Verification items for the finished model (mm, model axes). Give positions to 0.01 mm unless a question says otherwise; leave off trailing zeros. Order: outer loops, then holes, each group sorted by start corner. A loop starts at its lowest first (then second) coordinate and runs counter-clockwise, first axis right, second up. Notation, with made-up numbers: (45.5, -9.5) - (99.5, -9.5) arc R34 ccw to (99.5, 26.5) - close; hole circle Ø2 at (-14.5, -22). An arc over 180 degrees is marked (long way). Answer as a JSON object with one key per item and string values.
```python
from build123d import *

# Parameters (mm, degrees)
ESBO_O1_R                = 32
RESSALTO_EXTRUS_O1_DEPTH = 6
FURO_COM_FOLGA_DE_M51_D  = 5.5


with BuildPart() as part:
    # Esboço1 → Ressalto-extrusão1 (new body)
    with BuildSketch(Plane.XY.offset(10)):
        Polygon((16.091018061, 61.251677836), (45, 44.561069332), (45, -44.561069332), (16.091018061, -61.251677836), (-61.091018061, -16.690608504), (-61.091018061, 16.690608504), align=None)
        Circle(ESBO_O1_R, mode=Mode.SUBTRACT)
    extrude(amount=RESSALTO_EXTRUS_O1_DEPTH)

    # Furo com folga de M51 (through all)
    with Locations(Plane(origin=(-55, 0, 16), x_dir=(1, 0, 0), z_dir=(0, 0, 1))):
        with Locations((0, 0), (82.5, 47.631397208), (82.5, -47.631397208)):
            Hole(FURO_COM_FOLGA_DE_M51_D / 2)


solid = part.part
```
(1) Section check C-C (y = 21). Record the cut outline in (x, z).
Computed values:
{"outline": "(-53.63, 10) - (-24.15, 10) - (-24.15, 16) - (-53.63, 16) - close; (24.15, 10) - (45, 10) - (45, 16) - (24.15, 16) - close"}
(2) Gauge pin test, flat ends, axial feed: pin 1 Ø1 at (y, z) = (-30.5, 14) entering from -X; pin 2 Ø1.5 at (y, z) = (-24.5, 11) entering from -X. Record the tip position at first contact, or that the pin passes through.
Computed values:
{"pin 1": "stops at x = -38.04", "pin 2": "stops at x = -48.86"}
(3) Release check for a two-part mould opening along X. For faces 1 (the cylindrical face through (29.682, -49.305, 12.958)), 2 (the flat face through (45, 1, 13)), 3 (the flat face through (-19, -26, 10)) record: pulls with the +X half, pulls with the -X half, needs draft (parallel to the pull), parting line crosses it, or undercut.
Computed values:
{"face 1": "undercut", "face 2": "pulls with the +X half", "face 3": "needs draft"}
(4) Section check A-A (y = 0). Record the cut outline in (x, z).
Computed values:
{"outline": "(-61.09, 10) - (-57.75, 10) - (-57.75, 16) - (-61.09, 16) - close; (-52.25, 10) - (-32, 10) - (-32, 16) - (-52.25, 16) - close; (32, 10) - (45, 10) - (45, 16) - (32, 16) - close"}
(5) Section check D-D (z = 14.5). Record the cut outline in (x, y), then the cut area to 3 significant figures.
Computed values:
{"outline": "(-61.09, -16.69) - (16.09, -61.25) - (45, -44.56) - (45, 44.56) - (16.09, 61.25) - (-61.09, 16.69) - close; hole circle Ø5.5 at (-55, 0); hole circle Ø64 at (0, 0); hole circle Ø5.5 at (27.5, -47.63); hole circle Ø5.5 at (27.5, 47.63)", "area": "5,790 mm²"}
(6) Material ranges on line 1 along X through (y, z) = (0.5, 14.7); line 2 along X through (y, z) = (-2, 13.65); line 3 along Y through (x, z) = (27.5, 12), recorded low to high. Write a range as [from, to].
Computed values:
{"line 1": "x = [-61.09, -57.7], [-52.3, -32], [32, 45]", "line 2": "x = [-61.09, -56.89], [-53.11, -31.94], [31.94, 45]", "line 3": "y = [-54.66, -50.38], [-44.88, -16.36], [16.36, 44.88], [50.38, 54.66]"}
(7) Section check B-B (x = 0). Record the cut outline in (y, z), then the cut area to 3 significant figures.
Computed values:
{"outline": "(-51.96, 10) - (-32, 10) - (-32, 16) - (-51.96, 16) - close; (32, 10) - (51.96, 10) - (51.96, 16) - (32, 16) - close", "area": "240 mm²"}
